The model under review builds one solid part; all positions refer to its coordinate system, in mm. Face numbers are marked on the shaded views. A direction names the side the tool comes from. Round coordinates to 2 decimals unless told otherwise and drop trailing zeros. Order: outer loops, then holes, each group sorted by start corner. A loop starts at its lowest first (then second) coordinate and runs counter-clockwise, first axis right, second up. Notation, with made-up numbers: M -33.5,16 L 8.5,16 A21 cw 8.5,54 Z; hole C 59,89 d1. An arc over 180 degrees is marked long. Use a Markdown table: item, result. Add a question column.
1. Consider section A-A on z = 2.25. State the section outline as (x, y) points (1 decimal), then the cut area to 3 significant figures.
2. The part is to be moulded in two halves that separate along X. For the marked faces 4, 5 and 6, say which applies: +X half, -X half, draft (parallel to the pull), parting line (faces both ways), or undercut.
3. To check wall thickness, follow probe 1 along Y at (x, z) = (0, 12.8); probe 2 along Y at (x, z) = (-1.75, 12.75); probe 3 along X at (y, z) = (35.5, 1.5). State the ranges of each line that lie inside material, in increasing order.
4. Consider section B-B on y = 60. State the section outline as (x, z) points, then the cut area to 3 significant figures.
5. Insertion check: P1, Ø2, axis at y = 33.5, z = 10.5, coming from the +X side; P2, Ø5, axis at y = 54, z = 6, coming from the +X side; P3, Ø1, axis at x = -3, z = 1.5, coming from the +Y side. Each pin has a flat end and moves straight along its axis. Give the tip position at first contact, or say it passes through.
6. Consider section D-D on x = 0. State the section outline as (y, z) points.
7. For the marked faces 1, 2 and 3, list the 3-axis set-ups (+Z, -Z, +X, -X, +Y, -Y) from which the entire face can be reached by the end or side of a thin tool; tool diameter is ignored.
8. Consider section C-C on x = 4.75. State the section outline as (y, z) points, then the cut area to 3 significant figures.
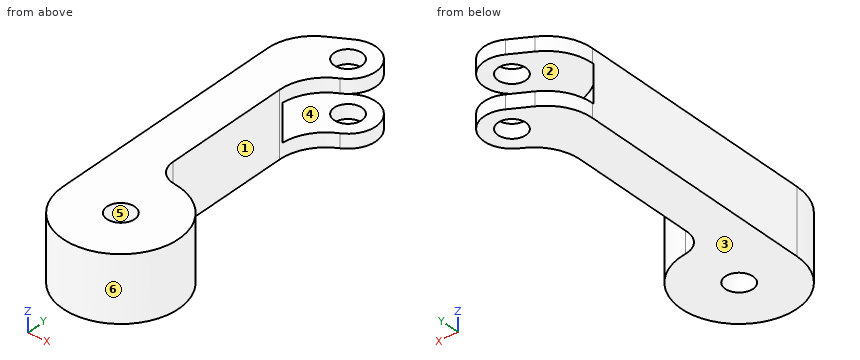
from build123d import *

# Parameters (mm, degrees)
CROQUIS1_R              = 3
SALIENTE_EXTRUIR1_DEPTH = 14
REDONDEO1_R             = 10
REDONDEO2_R             = 10
REDONDEO3_R             = 5
CORTAR_EXTRUIR1_START   = -3
CROQUIS2_R              = 14
CORTAR_EXTRUIR1_DEPTH   = 8


with BuildPart() as part:
    # Croquis1 → Saliente-Extruir1 (new body)
    with BuildSketch(Plane.XY):
        with BuildLine():
            ThreePointArc((-12.5, 0), (9.842509843, -7.705517504), (-3, 12.1346611))
            Line((-3, 12.1346611), (-3, 54.803847577))
            ThreePointArc((-3, 54.803847577), (5.999605182, 59.93116932), (-2.88, 65.263610928))
            Line((-2.88, 65.263610928), (-12.5, 60))
            Line((-12.5, 60), (-12.5, 0))
        make_face()
        Circle(CROQUIS1_R, mode=Mode.SUBTRACT)
        with Locations((0, 60)):
            Circle(CROQUIS1_R, mode=Mode.SUBTRACT)
    extrude(amount=SALIENTE_EXTRUIR1_DEPTH)

    # Redondeo1
    redondeo1_edges = [part.edges().sort_by_distance(p)[0] for p in [
        (-12.5, 60, 7),
    ]]
    fillet(redondeo1_edges, radius=REDONDEO1_R)

    # Redondeo2
    redondeo2_edges = [part.edges().sort_by_distance(p)[0] for p in [
        (-3, 54.803847577, 7),
    ]]
    fillet(redondeo2_edges, radius=REDONDEO2_R)

    # Redondeo3
    redondeo3_edges = [part.edges().sort_by_distance(p)[0] for p in [
        (-3, 12.1346611, 7),
    ]]
    fillet(redondeo3_edges, radius=REDONDEO3_R)

    # Croquis2 → Cortar-Extruir1 (cut)
    with BuildSketch(Plane.XY.offset(14).offset(CORTAR_EXTRUIR1_START)):
        with Locations((0, 60)):
            Circle(CROQUIS2_R)
    extrude(amount=-CORTAR_EXTRUIR1_DEPTH, mode=Mode.SUBTRACT)


solid = part.part
Answer block:
| question | item | result |
|---|---|---|
| 1 | outline | M -12.5,0 A12.5 ccw long 1.4,12.4 A5 cw -3,17.4 L -3,45.6 A10 cw 2.6,54.6 A6 ccw long -2.9,65.3 L -7.3,62.8 A10 ccw -12.5,54.1 Z; hole C 0,0 d6; hole C 0,60 d6 |
| 1 | area | 1,050 mm^2 |
| 2 | face 4 | draft |
| 2 | face 5 | undercut |
| 2 | face 6 | parting line |
| 3 | probe 1 | -12.5 to -3, 3 to 12.8, 52.75 to 57, 63 to 66 |
| 3 | probe 2 | -12.38 to -2.44, 2.44 to 14.08, 50.45 to 57.56, 62.44 to 65.74 |
| 3 | probe 3 | -12.5 to -3 |
| 4 | outline | M -10.55,0 L -3,0 L -3,3 L -10.55,3 Z; M -10.55,11 L -3,11 L -3,14 L -10.55,14 Z; M 3,0 L 6,0 L 6,3 L 3,3 Z; M 3,11 L 6,11 L 6,14 L 3,14 Z |
| 4 | area | 63.3 mm^2 |
| 5 | P1 | x = -3 |
| 5 | P2 | x = -11.12 |
| 5 | P3 | y = 65.45 |
| 6 | outline | M -12.5,0 L -3,0 L -3,14 L -12.5,14 Z; M 3,0 L 12.8,0 L 12.8,14 L 3,14 Z; M 52.75,0 L 57,0 L 57,3 L 52.75,3 Z; M 52.75,11 L 57,11 L 57,14 L 52.75,14 Z; M 63,0 L 66,0 L 66,3 L 63,3 Z; M 63,11 L 66,11 L 66,14 L 63,14 Z |
| 7 | face 1 | +Z, -Z, +X |
| 7 | face 2 | +X, +Y |
| 7 | face 3 | -Z, +X, -X, +Y, -Y |
| 8 | outline | M -11.56,0 L 11.56,0 L 11.56,14 L -11.56,14 Z; M 56.33,0 L 63.67,0 L 63.67,3 L 56.33,3 Z; M 56.33,11 L 63.67,11 L 63.67,14 L 56.33,14 Z |
| 8 | area | 368 mm^2 |
